Source: CAD feature listing. Evaluate the final solid. Frame: model axes, mm. Face numbers are marked on the shaded views. A direction names the side the tool comes from. Give positions to 0.01 mm unless a question says otherwise; leave off trailing zeros. Order: outer loops, then holes, each group sorted by start corner. A loop starts at its lowest first (then second) coordinate and runs counter-clockwise, first axis right, second up. Notation, with made-up numbers: (-17.5, 59) - (32.5, 59) arc R13 ccw to (32.5, 79) - close; hole circle Ø4 at (58, 38). An arc over 180 degrees is marked (long way). Use CSV: the item, a comma, the result in double quotes.
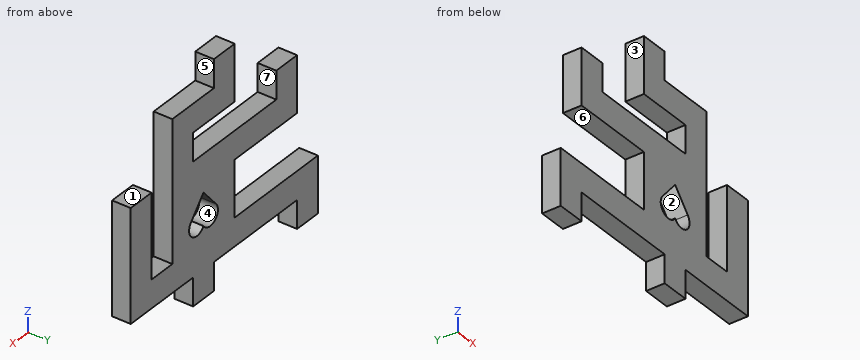
```python
from build123d import *

# Parameters (mm, degrees)
SKETCH1_W           = 22.5
SKETCH1_H           = 30
SKETCH1_W_2         = 7.5
SKETCH1_H_2         = 7.5
BOSS_EXTRUDE1_DEPTH = 5
CUT_EXTRUDE3_DEPTH  = 10


with BuildPart() as part:
    # Sketch1 → Boss-Extrude1 (new body)
    with BuildSketch(Plane(origin=(0, 0, 0), x_dir=(1, 0, 0), z_dir=(0, 1, 0))):
        Polygon((-11.25, 7.5), (-11.25, 15), (-33.75, 15), (-33.75, 22.5), (-41.25, 22.5), (-41.25, 7.5), align=None)
        Polygon((-26.25, -15), (-11.25, -15), (-11.25, -7.5), (-33.75, -7.5), (-33.75, -22.5), (-26.25, -22.5), align=None)
        Rectangle(SKETCH1_W, SKETCH1_H)
        Polygon((11.25, -30), (11.25, -15), (3.75, -15), (3.75, -22.5), (-11.25, -22.5), (-11.25, -37.5), (-3.75, -37.5), (-3.75, -30), align=None)
        with Locations((0, 18.75)):
            Rectangle(SKETCH1_W_2, SKETCH1_H_2)
        Polygon((26.25, 15), (11.25, 15), (11.25, 7.5), (18.75, 7.5), (18.75, -15), (26.25, -15), align=None)
    extrude(amount=BOSS_EXTRUDE1_DEPTH)

    # Sketch2 → Cut-Extrude3 (cut)
    with BuildSketch(Plane(origin=(0, 5, 0), x_dir=(1, 0, 0), z_dir=(0, 1, 0))):
        with BuildLine():
            Line((0, -5), (4.534880693, 0.371878565))
            ThreePointArc((4.534880693, 0.371878565), (4.042699073, 4.459844977), (0, 3.678630324))
            ThreePointArc((0, 3.678630324), (-4.042699073, 4.459844977), (-4.534880693, 0.371878565))
            Line((-4.534880693, 0.371878565), (0, -5))
        make_face()
    extrude(amount=-CUT_EXTRUDE3_DEPTH, mode=Mode.SUBTRACT)


solid = part.part
```
Item 1: Set-up query: the marked faces 5, 6 and 7. Return all of +Z, -Z, +X, -X, +Y, -Y with unobstructed straight access to the full face (end or side cutting, diameter ignored); none if empty.
Filled in:
face 5,"+Z, +X, +Y, -Y"
face 6,"-X, +Y, -Y"
face 7,"+Z, +Y, -Y"
Item 2: Section D-D on x = 1.5. Return the cut outline in (y, z).
Filled in:
outline,"(0, -22.5) - (5, -22.5) - (5, -4.86) - (0, -4.86) - close; (0, 3.22) - (5, 3.22) - (5, 15) - (0, 15) - close; (0, 22.5) - (5, 22.5) - (5, 30) - (0, 30) - close"
Item 3: Mould query, pull axis X, two halves, no side actions, for the marked faces 1, 2, 3 and 4. Classes: released by +X, released by -X, zero draft, split by the parting line, or undercut.
Filled in:
face 1,"zero draft"
face 2,"undercut"
face 3,"released by -X"
face 4,"undercut"
Item 4: Material intervals for line 1 (X direction, y = 1.95, z = -3); line 2 (Z direction, x = -27.5, y = 0.3); line 3 (Z direction, x = -21, y = 2.95), sorted ascending. Write a range as from..to.
Filled in:
line 1,"x = -11.25..-5.08, 5.08..11.25, 18.75..26.25"
line 2,"z = -15..-7.5, 7.5..22.5"
line 3,"z = -15..-7.5, 7.5..15"
Item 5: Section B-B on x = -7.5. Return the cut outline in (y, z).
Filled in:
outline,"(0, -15) - (5, -15) - (5, 15) - (0, 15) - close; (0, 22.5) - (5, 22.5) - (5, 37.5) - (0, 37.5) - close"
Item 6: First-contact query: pin 1 (2.5 mm diameter, centred on y = 2, z = -19.5, fed in from +X); pin 2 (1.5 mm diameter, centred on y = 1.5, z = 17.5, fed in from +X); pin 3 (2.5 mm diameter, centred on x = -24, y = 1.5, fed in from -Z). Flat tips, straight axial feed; report the tip coordinate or a pass-through.
Filled in:
pin 1,"stops at x = 3.75"
pin 2,"stops at x = 11.25"
pin 3,"stops at z = -15"
Item 7: Section A-A on z = 11. Return the cut outline in (x, y), then the cut area to 4 significant figures.
Filled in:
outline,"(-33.75, 0) - (11.25, 0) - (11.25, 5) - (-33.75, 5) - close; (18.75, 0) - (26.25, 0) - (26.25, 5) - (18.75, 5) - close"
area,"262.5 mm2"
